Autodesk Inventor part; units mm, degrees
ref_plane "YZ Plane" through (0, 0, 0) normal (1, 0, 0) x (0, 1, 0)
ref_plane "XZ Plane" through (0, 0, 0) normal (0, 1, 0) x (-1, 0, 0)
ref_plane "XY Plane" through (0, 0, 0) normal (0, 0, 1) x (1, 0, 0)
sketch "スケッチ1" plane through (0, 0, 0) normal (0, 0, 1) x (1, 0, 0)
  circle A0 centre (0, 0) radius 18.75
  circle A1 centre (0, 0) radius 20.5 construction
  circle A2 centre (0, 0) radius 20.51
  line L0 (0, 0) -> (0, 24.5) construction
  circle A3 centre (0, 24.5) radius 1.55
  circle A4 centre (0, 24.5) radius 3 construction
  arc A5 (0, 28.5) -> (-3.7147, 25.9835) centre (0, 24.5) ccw
  arc A6 (-5.1639, 24.7674) -> (-18.8673, 16.8557) centre (0, 0) ccw
  arc A7 (-5.1639, 24.7674) -> (-3.7147, 25.9835) centre (-5.5721, 26.7253) ccw
  arc A8 (3.7147, 25.9835) -> (0, 28.5) centre (0, 24.5) ccw
  arc A9 (3.7147, 25.9835) -> (5.1639, 24.7674) centre (5.5721, 26.7253) ccw
  circle A10 centre (0, 24.5) radius 3.05
  arc A11 (-24.0311, 7.9117) -> (-24.0311, -7.9117) centre (0, 0) ccw
  arc A12 (-24.0311, 7.9117) -> (-24.3598, 9.7747) centre (-25.9308, 8.5371) ccw
  arc A13 (-24.6817, 14.25) -> (-24.3598, 9.7747) centre (-21.2176, 12.25) ccw
  arc A14 (-20.645, 16.2088) -> (-24.6817, 14.25) centre (-21.2176, 12.25) ccw
  arc A15 (-20.645, 16.2088) -> (-18.8673, 16.8557) centre (-20.3588, 18.1882) ccw
  circle A16 centre (-21.2176, 12.25) radius 3.05
  circle A17 centre (-21.2176, 12.25) radius 1.55
  arc A18 (-18.8673, -16.8557) -> (-5.1639, -24.7674) centre (0, 0) ccw
  arc A19 (-18.8673, -16.8557) -> (-20.645, -16.2088) centre (-20.3588, -18.1882) ccw
  arc A20 (-24.6817, -14.25) -> (-20.645, -16.2088) centre (-21.2176, -12.25) ccw
  arc A21 (-24.3598, -9.7747) -> (-24.6817, -14.25) centre (-21.2176, -12.25) ccw
  arc A22 (-24.3598, -9.7747) -> (-24.0311, -7.9117) centre (-25.9308, -8.5371) ccw
  circle A23 centre (-21.2176, -12.25) radius 3.05
  circle A24 centre (-21.2176, -12.25) radius 1.55
  arc A25 (5.1639, -24.7674) -> (18.8673, -16.8557) centre (0, 0) ccw
  arc A26 (5.1639, -24.7674) -> (3.7147, -25.9835) centre (5.5721, -26.7253) ccw
  arc A27 (0, -28.5) -> (3.7147, -25.9835) centre (0, -24.5) ccw
  arc A28 (-3.7147, -25.9835) -> (0, -28.5) centre (0, -24.5) ccw
  arc A29 (-3.7147, -25.9835) -> (-5.1639, -24.7674) centre (-5.5721, -26.7253) ccw
  circle A30 centre (0, -24.5) radius 3.05
  circle A31 centre (0, -24.5) radius 1.55
  arc A32 (24.0311, -7.9117) -> (24.0311, 7.9117) centre (0, 0) ccw
  arc A33 (24.0311, -7.9117) -> (24.3598, -9.7747) centre (25.9308, -8.5371) ccw
  arc A34 (24.6817, -14.25) -> (24.3598, -9.7747) centre (21.2176, -12.25) ccw
  arc A35 (20.645, -16.2088) -> (24.6817, -14.25) centre (21.2176, -12.25) ccw
  arc A36 (20.645, -16.2088) -> (18.8673, -16.8557) centre (20.3588, -18.1882) ccw
  circle A37 centre (21.2176, -12.25) radius 3.05
  circle A38 centre (21.2176, -12.25) radius 1.55
  arc A39 (18.8673, 16.8557) -> (5.1639, 24.7674) centre (0, 0) ccw
  arc A40 (18.8673, 16.8557) -> (20.645, 16.2088) centre (20.3588, 18.1882) ccw
  arc A41 (24.6817, 14.25) -> (20.645, 16.2088) centre (21.2176, 12.25) ccw
  arc A42 (24.3598, 9.7747) -> (24.6817, 14.25) centre (21.2176, 12.25) ccw
  arc A43 (24.3598, 9.7747) -> (24.0311, 7.9117) centre (25.9308, 8.5371) ccw
  circle A44 centre (21.2176, 12.25) radius 3.05
  circle A45 centre (21.2176, 12.25) radius 1.55
  point P0 (-18.8673, 16.8557)
  point P1 (-24.0311, -7.9117)
  point P2 (-5.1639, -24.7674)
  point P3 (18.8673, -16.8557)
  point P4 (24.0311, 7.9117)
  dimension "d0" = 37.5
  dimension "d1" = 41
  dimension "d2" = 24.5
  dimension "d3" = 0.01
  dimension "d4" = 3.1
  dimension "d5" = 6
  dimension "d8" = 2
  dimension "d9" = 4.8
  dimension "d10" = 4
  dimension "d11" = 0.05
  dimension "d14" = 360
extrude "押し出し1" add sketch "スケッチ1" along normal blind 5 contours A8 A9 A39 A40 A41 A42 A43 A32 A33 A34 A35 A36 A25 A26 A27 A28 A29 A18 A19 A20 A21 A22 A11 A12 A13 A14 A15 A6 A7 A5
extrude "押し出し2" add sketch "スケッチ1" along normal blind 3.5 contours A2
extrude "押し出し3" add sketch "スケッチ1" along normal blind 2.5 contours A10 | A16 | A23 | A30 | A37 | A44
properties part number "Outer_support_stand" material "アルミニウム 2014-T4"
CAD build for the part. Positions are in the model's coordinates, mm. A direction names the side the tool comes from. Round coordinates to 2 decimals unless told otherwise and drop trailing zeros. Order: outer loops, then holes, each group sorted by start corner. A loop starts at its lowest first (then second) coordinate and runs counter-clockwise, first axis right, second up. Notation, with made-up numbers: M -23.75,29 L 32.25,29 A12 cw 32.25,45 Z; hole C -15,72.5 d5. An arc over 180 degrees is marked long. Use one line per item in the form item = value.
Q1. Saw through at A-A on y = 0. Give the cut face in (x, z), then the cut area to 3 significant figures.
Recorded:
outline = M -25.3,0 L -18.75,0 L -18.75,3.5 L -20.51,3.5 L -20.51,5 L -25.3,5 Z; M 18.75,0 L 25.3,0 L 25.3,5 L 20.51,5 L 20.51,3.5 L 18.75,3.5 Z
area = 60.2 mm^2
Q2. Saw through at D-D on x = -21.5. Give the cut face in (y, z), then the cut area to 3 significant figures.
Recorded:
outline = M -16.24,0 L -13.77,0 L -13.77,2.5 L -15.29,2.5 L -15.29,5 L -16.24,5 Z; M -10.73,0 L 10.73,0 L 10.73,2.5 L 9.21,2.5 L 9.21,5 L -9.21,5 L -9.21,2.5 L -10.73,2.5 Z; M 13.77,0 L 16.24,0 L 16.24,5 L 15.29,5 L 15.29,2.5 L 13.77,2.5 Z
area = 117 mm^2
Q3. Probe L1, parallel to Y at x = 0, z = 2.55; L2, parallel to Y at x = 0.5, z = 0.35; L3, parallel to Y at x = 23, z = 4.3. List the from-to ranges inside material, lowest first.
Recorded:
L1 = -28.5 to -27.55, -21.45 to -18.75, 18.75 to 21.45, 27.55 to 28.5
L2 = -28.47 to -25.97, -23.03 to -18.74, 18.74 to 23.03, 25.97 to 28.47
L3 = -15.83 to -14.72, -9.78 to 9.78, 14.72 to 15.83
Q4. Saw through at C-C on y = 12.25. Give the cut face in (x, z), then the cut area to 3 significant figures.
Recorded:
outline = M -25.22,0 L -22.77,0 L -22.77,2.5 L -24.27,2.5 L -24.27,5 L -25.22,5 Z; M -19.67,0 L -14.2,0 L -14.2,3.5 L -16.45,3.5 L -16.45,5 L -18.17,5 L -18.17,2.5 L -19.67,2.5 Z; M 14.2,0 L 19.67,0 L 19.67,2.5 L 18.17,2.5 L 18.17,5 L 16.45,5 L 16.45,3.5 L 14.2,3.5 Z; M 22.77,0 L 25.22,0 L 25.22,5 L 24.27,5 L 24.27,2.5 L 22.77,2.5 Z
area = 57.5 mm^2
Q5. Two-plate mould, pull along Y, no slides. Class faces 3 (the cylindrical face through (-2.271, 27.793, 2.465)), 4 (the cylindrical face through (-22.766, -12.318, 1.232)), 5 (the cylindrical face through (22.994, -15.834, 2.465)): +Y half, -Y half, draft (parallel to the pull), parting line (faces both ways), or undercut.
Recorded:
face_3 = +Y half
face_4 = undercut
face_5 = -Y half
Q6. Flat gauge pins, fed straight in: P1, Ø1.9, axis at x = -21.22, y = -12.25, coming from the +Z side; P2, Ø5, axis at x = 21.5, y = 12, coming from the +Z side. Where does each tip first touch, or does it go through?
Recorded:
P1 = through
P2 = 2.5
Q7. Which spindle directions (+Z, -Z, +X, -X, +Y, -Y) get a long thin tool onto all of the face, cutting with end or side? Do faces 1 (the flat face through (9, -17, 3.5)), 2 (the cylindrical face through (-25.205, 11.93, 2.465)). Say none if no direction does.
Recorded:
face_1 = +Z
face_2 = +Z, -Z, -X
Q8. Saw through at B-B on x = 11.5. Give the cut face in (y, z).
Recorded:
outline = M -22.54,0 L -14.81,0 L -14.81,3.5 L -16.98,3.5 L -16.98,5 L -22.54,5 Z; M 14.81,0 L 22.54,0 L 22.54,5 L 16.98,5 L 16.98,3.5 L 14.81,3.5 Z
